Print and shaded views of the part. All mm, measured from the part's lowest x, y and z. A direction names the side the tool comes from. Coordinates: 2 decimals unless noted, no trailing zeros. Order: outer loops, then holes, each group sorted by start corner. A loop starts at its lowest first (then second) coordinate and runs counter-clockwise, first axis right, second up. Notation, with made-up numbers: M 11.25,41 L 17.25,41 A8 ccw 17.25,53 Z; hole C 45.5,43.5 d1. An arc over 180 degrees is marked long. Return JSON: item names as keys, results as strings.
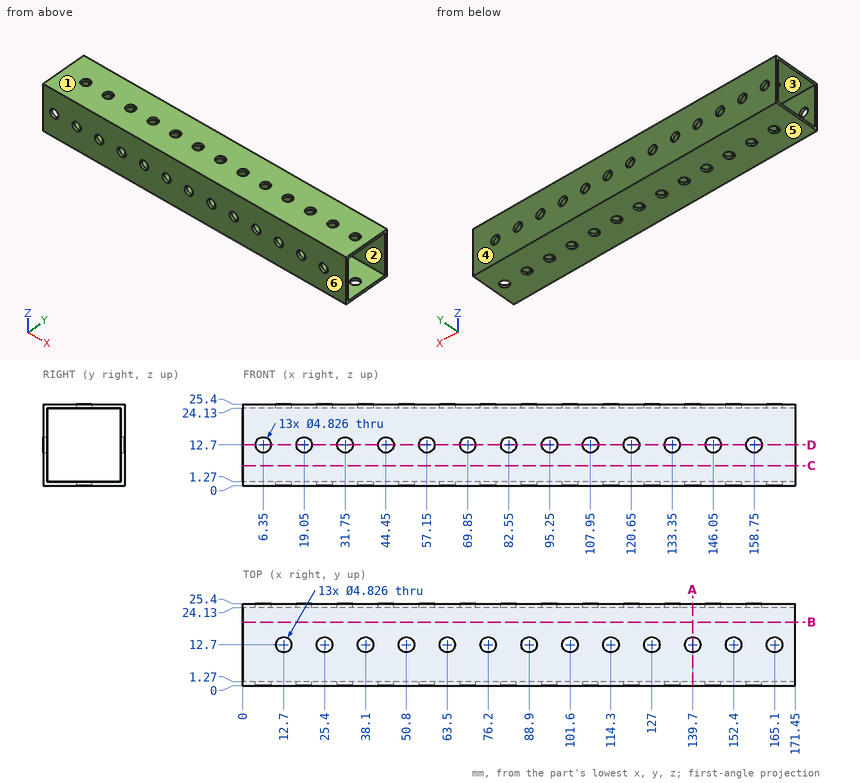
Item 1: Saw through at D-D (z = 12.7). Count the separate pieces of the cut face and the enclosed holes in it, and give its area (3 significant figures).
Check result:
{"separate pieces": "28", "enclosed holes": "0", "area": "276 mm2"}
Item 2: Drop a flat-ended pin along its axis: pin 1 Ø10 at (y, z) = (10.5, 15) entering from -X. Give the stop position or say it passes through.
Check result:
{"pin 1": "passes through"}
Item 3: Pull direction Y, two halves, no side cores. Call the marked faces 3, 4, 5 and 6: +Y half, -Y half, draft (parallel to the pull), parting line (faces both ways), or undercut.
Check result:
{"face 3": "undercut", "face 4": "+Y half", "face 5": "draft", "face 6": "-Y half"}
Item 4: Wall check: line 1 (Z direction, x = 114, y = 23); line 2 (Y direction, x = 88.9, z = 0.9). Give the ranges that are in metal, low to high.
Check result:
{"line 1": "z = 0 to 1.27, 24.13 to 25.4", "line 2": "y = 0 to 10.29, 15.11 to 25.4"}
Item 5: 3-axis set-ups, long thin cutter, end or side, ignore diameter. For the marked faces 1 and 2: which of +Z, -Z, +X, -X, +Y, -Y reach the whole face in a straight line?
Check result:
{"face 1": "+Z, +X, -X, +Y, -Y", "face 2": "+X, -X"}
Item 6: Saw through at A-A (x = 139.7). Write the cut outline in (y, z).
Check result:
{"outline": "M 0,0 L 10.29,0 L 10.29,1.27 L 1.27,1.27 L 1.27,24.13 L 10.29,24.13 L 10.29,25.4 L 0,25.4 Z; M 15.11,0 L 25.4,0 L 25.4,25.4 L 15.11,25.4 L 15.11,24.13 L 24.13,24.13 L 24.13,1.27 L 15.11,1.27 Z"}
Item 7: Saw through at B-B (y = 19.75). Write the cut outline in (x, z), and give its area (3 significant figures).
Check result:
{"outline": "M 0,0 L 171.45,0 L 171.45,1.27 L 0,1.27 Z; M 0,24.13 L 171.45,24.13 L 171.45,25.4 L 0,25.4 Z", "area": "435 mm2"}
